The listing builds one solid part. Answer for the finished solid, in the listing's coordinates (mm). Face numbers are marked on the shaded views. A direction names the side the tool comes from. Coordinates: 2 decimals unless noted, no trailing zeros. Order: outer loops, then holes, each group sorted by start corner. A loop starts at its lowest first (then second) coordinate and runs counter-clockwise, first axis right, second up. Notation, with made-up numbers: (4, 70) -> (60, 70) arc R25 cw to (60, 98) -> close; hole circle Ø11 at (8.25, -37.75). An arc over 180 degrees is marked (long way). Return JSON: item names as keys, results as strings.
from build123d import *

# Parameters (mm, degrees)
F0_W     = 36.3202914596
F0_H     = 46.1400337517
F1_DEPTH = 8.89
F3_DEPTH = 6.985
F5_DEPTH = 25.4
F6_DEPTH = 6.35
F7_DEPTH = 6.096


with BuildPart() as f1:
    # F0 (on Top) → F1 (new body)
    with BuildSketch(Plane.XY):
        with Locations((18.1601457298, -23.0700168759)):
            Rectangle(F0_W, F0_H)
    extrude(amount=F1_DEPTH)

    # F2 (on face) → F3 (cut)
    with BuildSketch(Plane.XY.offset(8.89)):
        with BuildLine():
            Line((11.814377988, -29.4157846176), (24.5059134716, -29.4157846176))
            ThreePointArc((24.5059134716, -29.4157846176), (30.8516812133, -23.0700168759), (24.5059134716, -16.7242491341))
            Line((24.5059134716, -16.7242491341), (11.814377988, -16.7242491341))
            ThreePointArc((11.814377988, -16.7242491341), (5.4686102462, -23.0700168759), (11.814377988, -29.4157846176))
        make_face()
    extrude(amount=-F3_DEPTH, mode=Mode.SUBTRACT)

    # F4 (on face) → F5 (join)
    with BuildSketch(Plane(origin=(0, 0, 0), x_dir=(-1, 0, 0), z_dir=(0, 1, 0))):
        Polygon((-24.5190151036, 0), (-11.8220960721, 0), (-11.8220960721, 4.445), (-11.8220960721, 8.89), (-24.5190151036, 8.89), (-24.5190151036, 4.445), align=None)
    extrude(amount=F5_DEPTH)

    # F6 (cut): a face of the model
    f6_faces = [f1.faces().sort_by_distance(p)[0] for p in [
        (18.1601457298, -46.1400337517, 4.445),
    ]]
    extrude(f6_faces, amount=-F6_DEPTH, mode=Mode.SUBTRACT)

    # F7 (cut): faces of the model
    f7_faces = [f1.faces().sort_by_distance(p)[0] for p in [
        (5.9110480361, 0, 4.445),
        (30.4196532816, 0, 4.445),
    ]]
    extrude(f7_faces, amount=-F7_DEPTH, mode=Mode.SUBTRACT)


solid = f1.part
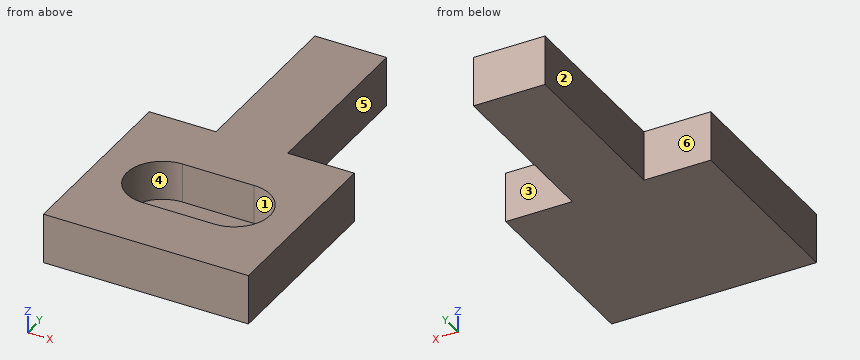
1. For the marked faces 1, 2 and 3, determine the directions among +Z, -Z, +X, -X, +Y, -Y from which every point of the face is accessible in a straight line to the end or side of a thin tool.
Answer block:
{"face 1": "+Z", "face 2": "+Z, -Z, -X, +Y", "face 3": "+Z, -Z, +X, +Y"}
2. Each of these flat-tipped pins is pushed along its axis until it touches: pin 1 Ø5 at (y, z) = (14.5, 8) entering from -X; pin 2 Ø2.5 at (y, z) = (5, 6.5) entering from +X; pin 3 Ø1.5 at (x, z) = (6, 6) entering from +Y. Where does it stop, or does it pass through?
Answer block:
{"pin 1": "stops at x = 11.82", "pin 2": "stops at x = 24.52", "pin 3": "stops at y = -6.1"}
3. The part is cut by section C-C on y = 18. Give the vertices of the cut face in (x, z).
Answer block:
{"outline": "(11.82, 0) -> (24.52, 0) -> (24.52, 8.89) -> (11.82, 8.89) -> close"}
4. Consider line 1 (Y direction, x = 17.5, z = 2.75); line 2 (X direction, y = -4, z = 4); line 3 (Y direction, x = 31, z = 8). Determine where each line is inside the solid, lowest interval first. Write a range as from..to.
Answer block:
{"line 1": "y = -39.79..-29.42, -16.72..25.4", "line 2": "x = 11.82..24.52", "line 3": "y = -39.79..-6.1"}
5. The part is cut by section D-D on x = 30. Give the vertices of the cut face in (y, z) (3 decimals), and give its area (3 significant figures).
Answer block:
{"outline": "(-39.79, 0) -> (-6.096, 0) -> (-6.096, 8.89) -> (-19.895, 8.89) -> (-19.895, 1.905) -> (-26.246, 1.905) -> (-26.246, 8.89) -> (-39.79, 8.89) -> close", "area": "255 mm2"}
6. Determine the mould class of the marked faces 4, 5 and 6 for opening direction X: pulls with the +X half, pulls with the -X half, needs draft (parallel to the pull), parting line crosses it, or undercut.
Answer block:
{"face 4": "undercut", "face 5": "pulls with the +X half", "face 6": "needs draft"}
7. The part is cut by section A-A on z = 7.25. Give the vertices of the cut face in (x, y).
Answer block:
{"outline": "(0, -39.79) -> (36.32, -39.79) -> (36.32, -6.1) -> (24.52, -6.1) -> (24.52, 25.4) -> (11.82, 25.4) -> (11.82, -6.1) -> (0, -6.1) -> close; hole (11.81, -29.42) -> (24.51, -29.42) arc R6.35 ccw to (24.51, -16.72) -> (11.81, -16.72) arc R6.35 ccw to start"}
8. The part is cut by section B-B on x = 18.5. Give the vertices of the cut face in (y, z) (3 decimals).
Answer block:
{"outline": "(-39.79, 0) -> (25.4, 0) -> (25.4, 8.89) -> (-16.724, 8.89) -> (-16.724, 1.905) -> (-29.416, 1.905) -> (-29.416, 8.89) -> (-39.79, 8.89) -> close"}
